Autodesk Inventor part; units mm, degrees
ref_plane "YZ Plane" through (0, 0, 0) normal (1, 0, 0) x (0, 1, 0)
ref_plane "XZ Plane" through (0, 0, 0) normal (0, 1, 0) x (-1, 0, 0)
ref_plane "XY Plane" through (0, 0, 0) normal (0, 0, 1) x (1, 0, 0)
sketch "Sketch1" plane through (0, 0, 0) normal (0, 1, 0) x (-1, 0, 0)
  line L0 (-38.1, 63.5) -> (38.1, 63.5)
  line L1 (38.1, 63.5) -> (38.1, -63.5)
  line L2 (38.1, -63.5) -> (-38.1, -63.5)
  line L3 (-38.1, -63.5) -> (-38.1, 63.5)
  line L4 (-38.1, 63.5) -> (38.1, -63.5) construction
  line L5 (38.1, 63.5) -> (-38.1, -63.5) construction
  line L6 (-31.75, -50.8) -> (31.75, -50.8)
  line L7 (31.75, -50.8) -> (31.75, 50.8)
  line L8 (31.75, 50.8) -> (-31.75, 50.8)
  line L9 (-31.75, 50.8) -> (-31.75, -50.8)
  line L10 (-31.75, -50.8) -> (31.75, 50.8) construction
  line L11 (31.75, -50.8) -> (-31.75, 50.8) construction
  point P0 (0, 0)
  dimension "d0" = 76.2
  dimension "d1" = 127
  dimension "d2" = 63.5
  dimension "d3" = 101.6
extrude "Extrusion1" add sketch "Sketch1" along normal blind 25.4
sketch "Sketch2" plane through (0, 0, 0) normal (0, -1, 0) x (1, 0, 0)
  line L0 (-38.1, 63.5) -> (38.1, 63.5)
  line L1 (38.1, -63.5) -> (-38.1, -63.5)
  line L2 (38.1, 63.5) -> (-38.1, 63.5)
  line L3 (-38.1, 63.5) -> (-38.1, -63.5)
  line L4 (-38.1, -63.5) -> (38.1, -63.5)
  line L5 (38.1, -63.5) -> (38.1, 63.5)
  point P0 (0, 0)
extrude "Extrusion2" add sketch "Sketch2" along normal blind 6.35
fillet "Fillet1" radius 5.08 4 edges at (38.1, -6.35, 0) (0, -6.35, -63.5) (-38.1, -6.35, 0) (0, -6.35, 63.5)
fillet "Fillet2" radius 5.08 8 edges at (36.6121, -4.8621, -62.0121) (38.1, 12.065, -63.5) (-36.6121, -4.8621, -62.0121) (-38.1, 12.065, -63.5) (36.6121, -4.8621, 62.0121) (38.1, 12.065, 63.5) (-36.6121, -4.8621, 62.0121) (-38.1, 12.065, 63.5)
sketch "Sketch3" plane through (0, 0, 0) normal (0, 1, 0) x (1, 0, 0)
  circle A0 centre (0, 0) radius 14.5196
extrude "Extrusion3" add sketch "Sketch3" along normal up to surface (25.4 mm away)
properties part number "TestPart"
Read the model definition and answer for the solid it produces. Units are mm, in the model's axes. A direction names the side the tool comes from. Coordinates: 2 decimals unless noted, no trailing zeros. Loops run counter-clockwise (first coordinate to the right, second up) from the corner with the lowest first, then second, coordinate; pieces in that order, holes last.
Q1. The part is cut by section A-A on y = 12.5. Write down the section's boundary in (x, z).
Q2. The part is cut by section B-B on x = -21. Write down the section's boundary in (y, z), and give its area (3 significant figures).
Q3. Consider probe 1 along X at (y, z) = (6, 0); probe 2 along X at (y, z) = (23, -46); probe 3 along Z at (x, y) = (19.5, 1). Determine where each line is inside the solid, lowest interval first.
Q4. The part is cut by section D-D on z = 16.5. Write down the section's boundary in (x, y), and give its area (3 significant figures).
Q5. The mould has two halves that part along X. Classify faces 3 (the face through (-31.75, 13, -1)), 4 (the face through (36.572, 11.878, -62.051)), 5 (the face through (-38.1, 12, 1)): +X half, -X half, draft (parallel to the pull), parting line (faces both ways), or undercut.
Q6. Which of the six approach directions +Z, -Z, +X, -X, +Y, -Y give full straight-line access (tool end or side, diameter ignored) to faces 1 (the face through (0, 13, 50.8)), 2 (the face through (-0.462, -4.822, -62.051))?
Q7. This flat-tipped pin is pushed along its axis until it touches: pin 1 Ø5 at (x, z) = (27.5, -13) entering from +Y. Where does it stop, or does it pass through?
Q8. The part is cut by section C-C on z = 0. Write down the section's boundary in (x, y).
Results below:
1. outline: (-38.1, -58.42) arc R5.08 ccw to (-33.02, -63.5) - (33.02, -63.5) arc R5.08 ccw to (38.1, -58.42) - (38.1, 58.42) arc R5.08 ccw to (33.02, 63.5) - (-33.02, 63.5) arc R5.08 ccw to (-38.1, 58.42) - close; circle Ø29.04 at (0, 0); hole (-31.75, -50.8) - (31.75, -50.8) - (31.75, 50.8) - (-31.75, 50.8) - close
2. outline: (-6.35, -58.42) arc R5.08 ccw to (-1.27, -63.5) - (25.4, -63.5) - (25.4, -50.8) - (0, -50.8) - (0, 50.8) - (25.4, 50.8) - (25.4, 63.5) - (-1.27, 63.5) arc R5.08 ccw to (-6.35, 58.42) - close
2. area: 1,440 mm2
3. probe 1: x = -38.1 to -31.75, -14.52 to 14.52, 31.75 to 38.1
3. probe 2: x = -38.1 to -31.75, 31.75 to 38.1
3. probe 3: z = -63.5 to -50.8, 50.8 to 63.5
4. outline: (-38.1, -1.27) arc R5.08 ccw to (-33.02, -6.35) - (33.02, -6.35) arc R5.08 ccw to (38.1, -1.27) - (38.1, 25.4) - (31.75, 25.4) - (31.75, 0) - (-31.75, 0) - (-31.75, 25.4) - (-38.1, 25.4) - close
4. area: 795 mm2
5. face 3: undercut
5. face 4: +X half
5. face 5: -X half
6. face 1: +Y
6. face 2: -Z, +X, -X, -Y
7. pin 1: stops at y = 0
8. outline: (-38.1, -1.27) arc R5.08 ccw to (-33.02, -6.35) - (33.02, -6.35) arc R5.08 ccw to (38.1, -1.27) - (38.1, 25.4) - (31.75, 25.4) - (31.75, 0) - (14.52, 0) - (14.52, 25.4) - (-14.52, 25.4) - (-14.52, 0) - (-31.75, 0) - (-31.75, 25.4) - (-38.1, 25.4) - close
